```python
from build123d import *

# Parameters (mm, degrees)
EXTRUDE1_DEPTH = 3.175
SKETCH2_R      = 2.0701
EXTRUDE2_DEPTH = 200.886360684
SKETCH3_R      = 6.35
EXTRUDE3_DEPTH = 200.886360684


with BuildPart() as part:
    # Sketch1 → Extrude1 (new body)
    with BuildSketch(Plane(origin=(0, 0, 0), x_dir=(1, 0, 0), z_dir=(0, 1, 0))):
        Polygon((-138.1125, 144.4625), (138.1125, 144.4625), (138.1125, -70.2437), (51.1937, -70.2437), (51.1937, -144.4625), (-138.1125, -144.4625), align=None)
        Polygon((-125.0188, 131.3688), (125.0188, 131.3688), (125.0188, -57.15), (38.1, -57.15), (38.1, -131.3688), (-125.0188, -131.3688), align=None, mode=Mode.SUBTRACT)
    extrude(amount=EXTRUDE1_DEPTH)

    # Sketch2 → Extrude2 (cut, through all)
    with BuildSketch(Plane(origin=(0, 3.175, 0), x_dir=(-1, 0, 0), z_dir=(0, 1, 0))):
        with Locations(Location((24.13, 139.446, 0), (0, 0, 90))):
            Circle(SKETCH2_R)
        with Locations(Location((104.775, -139.446, 0), (0, 0, 90))):
            Circle(SKETCH2_R)
        with Locations(Location((3.175, -139.446, 0), (0, 0, 90))):
            Circle(SKETCH2_R)
        with Locations(Location((133.096, 104.9365694, 0), (0, 0, 90))):
            Circle(SKETCH2_R)
        with Locations(Location((133.096, 3.3365694, 0), (0, 0, 90))):
            Circle(SKETCH2_R)
        with Locations(Location((133.096, -98.2634306, 0), (0, 0, 90))):
            Circle(SKETCH2_R)
        with Locations(Location((-98.425, -139.446, 0), (0, 0, 90))):
            Circle(SKETCH2_R)
        with Locations(Location((-133.096, -76.2, 0), (0, 0, 90))):
            Circle(SKETCH2_R)
        with Locations(Location((-133.096, 12.7, 0), (0, 0, 90))):
            Circle(SKETCH2_R)
        with Locations(Location((-46.1772, 82.55, 0), (0, 0, 90))):
            Circle(SKETCH2_R)
    extrude(amount=-EXTRUDE2_DEPTH, mode=Mode.SUBTRACT)

    # Sketch3 → Extrude3 (cut, through all)
    with BuildSketch(Plane(origin=(0, 3.175, 0), x_dir=(-1, 0, 0), z_dir=(0, 1, 0))):
        with Locations((69.99986, 145.00098)):
            Circle(SKETCH3_R)
        with Locations((69.99986, -145.00098)):
            Circle(SKETCH3_R)
        with Locations((-69.99986, -145.00098)):
            Circle(SKETCH3_R)
    extrude(amount=-EXTRUDE3_DEPTH, mode=Mode.SUBTRACT)


solid = part.part
```
Can you work these out from the model? Positions are in its coordinate system, mm. Round coordinates to 2 decimals unless told otherwise and drop trailing zeros. Loops run counter-clockwise (first coordinate to the right, second up) from the corner with the lowest first, then second, coordinate; pieces in that order, holes last.
Item 1: Suppose I cut it at C-C, the plane y = 1.4. State how many separate pieces and enclosed holes the cut face has, then the cut area to 3 significant figures.
Item 2: Suppose I cut it at B-B, the plane x = -118. Write out the boundary of the cut face in (y, z) (1 decimal), then the cut area to 3 significant figures.
Item 3: Please list where these lines run through material, in increasing order: L1, parallel to X at y = 1.65, z = -76.2; L2, parallel to X at y = 2.6, z = 7.5; L3, parallel to Z at x = 19.5, y = 1.4.
Item 4: Will this pin go through, and if not, where does the flat tip stop? pin 1 Ø1 at (x, y) = (106, 1.5) entering from +Z.
Item 5: Suppose I cut it at A-A, the plane z = 25. Write out the boundary of the cut face in (x, y) (1 decimal).
Reported:
1. separate pieces: 1
1. enclosed holes: 11
1. area: 13,800 mm2
2. outline: (0, -144.5) - (3.2, -144.5) - (3.2, -131.4) - (0, -131.4) - close; (0, 131.4) - (3.2, 131.4) - (3.2, 144.5) - (0, 144.5) - close
2. area: 83.1 mm2
3. L1: x = -138.11 to -125.02, 125.02 to 131.03, 135.17 to 138.11
3. L2: x = -138.11 to -125.02, 125.02 to 138.11
3. L3: z = -144.46 to -131.37, 131.37 to 144.46
4. pin 1: stops at z = 70.24
5. outline: (-138.1, 0) - (-125, 0) - (-125, 3.2) - (-138.1, 3.2) - close; (125, 0) - (138.1, 0) - (138.1, 3.2) - (125, 3.2) - close
